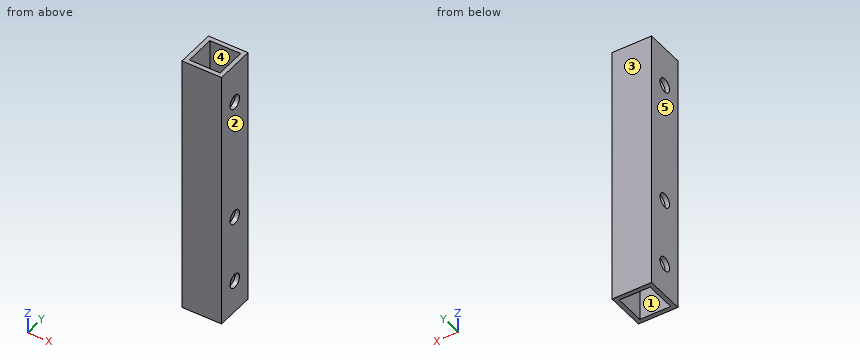
Autodesk Inventor part; units mm, degrees
ref_plane "YZ Plane" through (0, 0, 0) normal (1, 0, 0) x (0, 1, 0)
ref_plane "XZ Plane" through (0, 0, 0) normal (0, 1, 0) x (-1, 0, 0)
ref_plane "XY Plane" through (0, 0, 0) normal (0, 0, 1) x (1, 0, 0)
sketch "スケッチ1" plane through (0, 0, 0) normal (0, 0, 1) x (1, 0, 0)
  line L0 (4.5, 4.5) -> (-4.5, 4.5)
  line L1 (-4.5, 4.5) -> (-4.5, -4.5)
  line L2 (-4.5, -4.5) -> (4.5, -4.5)
  line L3 (4.5, -4.5) -> (4.5, 4.5)
  line L4 (4.5, 4.5) -> (-4.5, -4.5) construction
  line L5 (-4.5, 4.5) -> (4.5, -4.5) construction
  line L6 (-3.5, 3.5) -> (3.5, 3.5)
  line L7 (3.5, 3.5) -> (3.5, -3.5)
  line L8 (3.5, -3.5) -> (-3.5, -3.5)
  line L9 (-3.5, -3.5) -> (-3.5, 3.5)
  point P0 (0, 0)
  dimension "d0" = 9
  dimension "d1" = 9
  dimension "d2" = 1
extrude "押し出し1" add sketch "スケッチ1" along normal blind 60
sketch "スケッチ2" plane through (4.5, -4.5, 0) normal (1, 0, 0) x (0, 0, -1)
  circle A0 centre (-7.5, 4.5) radius 1.6
  circle A1 centre (-23, 4.5) radius 1.6
  circle A2 centre (-51, 4.5) radius 1.6
  line L0 (0, 0) -> (0, 9)
  point P0 (0, 4.5)
  point P1 (0, 4.5)
  dimension "d5" = 3.2
  dimension "d6" = 3.2
  dimension "d7" = 3.2
  dimension "d9" = 7.5
  dimension "d11" = 15.5
  dimension "d12" = 28
extrude "押し出し2" cut sketch "スケッチ2" against normal through all
properties part number "ハンド_角柱1" material "アルミニウム 6061"
Source: CAD feature listing. Evaluate the final solid. Frame: model axes, mm. Face numbers are marked on the shaded views. A direction names the side the tool comes from. Give positions to 0.01 mm unless a question says otherwise; leave off trailing zeros. Write each loop counter-clockwise with the first axis right and the second up, starting at its lowest first coordinate (ties: lowest second). Pieces come first, ordered by that corner, then holes. Notation, with made-up numbers: (-27.75, 53) -> (27.25, 53) arc R14 cw to (27.25, 64) -> close; hole circle Ø6 at (86, 47.25). An arc over 180 degrees is marked (long way). Return JSON: item names as keys, results as strings. Group by question number.
1. Section A-A, the plane x = 1. Output: boundary loops of the cut face in (y, z).
2. Material intervals for line 1 (Y direction, x = -3.9, z = 51); line 2 (X direction, y = -2.75, z = 47), sorted ascending. Write a range as from..to.
3. Section C-C, the plane y = 0. Count the separate pieces of the cut face and the enclosed holes in it, then the cut area to 3 significant figures.
4. Access query for the marked faces 4 and 5. Directions: +Z, -Z, +X, -X, +Y, -Y. A direction counts if a zero-diameter tool reaches every point of the face in a straight line with its end or side. Return the directions, or none.
5. Section D-D, the plane z = 55.5. Output: boundary loops of the cut face in (x, y).
6. Mould query, pull axis X, two halves, no side actions, for the marked faces 1, 2 and 3. Classes: +X half, -X half, draft (parallel to the pull), parting line (faces both ways), or undercut.
7. Section B-B, the plane z = 23. Output: boundary loops of the cut face in (x, y).
8. Pin query (flat end, axial travel): pin 1 Ø2.5 at (y, z) = (0, 51) entering from -X; pin 2 Ø3.5 at (y, z) = (0, 7.5) entering from +X. Return the tip coordinate at first contact, or that it passes through.
Determined:
{
 "1": {"outline": "(-4.5, 0) -> (-3.5, 0) -> (-3.5, 60) -> (-4.5, 60) -> close; (3.5, 0) -> (4.5, 0) -> (4.5, 60) -> (3.5, 60) -> close"},
 "2": {"line 1": "y = -4.5..-1.6, 1.6..4.5", "line 2": "x = -4.5..-3.5, 3.5..4.5"},
 "3": {"separate pieces": "8", "enclosed holes": "0", "area": "101 mm2"},
 "4": {"face 4": "+Z, -Z", "face 5": "+Z, -Z, -X, +Y, -Y"},
 "5": {"outline": "(-4.5, -4.5) -> (4.5, -4.5) -> (4.5, 4.5) -> (-4.5, 4.5) -> close; hole (-3.5, -3.5) -> (3.5, -3.5) -> (3.5, 3.5) -> (-3.5, 3.5) -> close"},
 "6": {"face 1": "undercut", "face 2": "+X half", "face 3": "draft"},
 "7": {"outline": "(-4.5, -4.5) -> (4.5, -4.5) -> (4.5, -1.6) -> (3.5, -1.6) -> (3.5, -3.5) -> (-3.5, -3.5) -> (-3.5, -1.6) -> (-4.5, -1.6) -> close; (-4.5, 1.6) -> (-3.5, 1.6) -> (-3.5, 3.5) -> (3.5, 3.5) -> (3.5, 1.6) -> (4.5, 1.6) -> (4.5, 4.5) -> (-4.5, 4.5) -> close"},
 "8": {"pin 1": "passes through", "pin 2": "stops at x = 4.5"}
}
